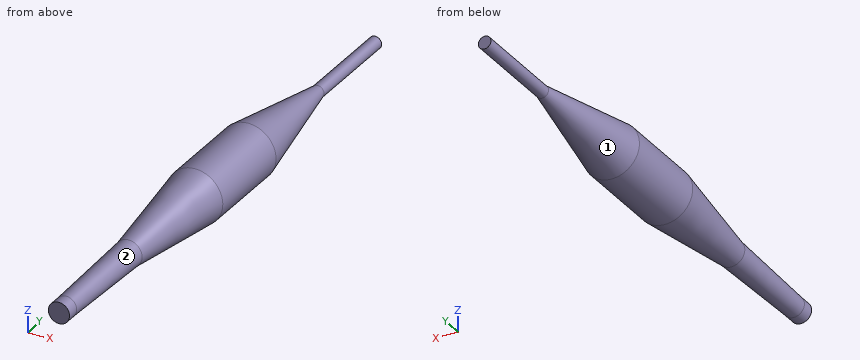
from build123d import *

# Parameters (mm, degrees)
F0_W   = 25
F0_H   = 21
F0_W_2 = 184.9109574539
F0_H_2 = 55
F0_W_3 = 200
F0_H_3 = 12.5


# Not quite as in the source:
# - the program builds the solid bodies; features that only make, move or delete a surface that nothing else refers to are left out


with BuildPart() as f1:
    # F0 (on Right) → F1 (revolve)
    with BuildSketch(Plane.YZ):
        with Locations((12.5, 223.4762815751)):
            Rectangle(F0_W, F0_H)
        Polygon((25, 233.9762815751), (25, 212.9762815751), (242, 212.9762815751), (242, 239.6586265556), align=None)
        Polygon((242, 239.6586265556), (242, 212.9762815751), (344.0616714118, 212.9762815751), (344.0616714118, 252.1902240649), align=None)
        Polygon((344.0616714118, 252.1902240649), (344.0616714118, 212.9762815751), (472.6287925066, 212.9762815751), (472.6287925066, 267.9762815751), align=None)
        with Locations((565.0842712335, 240.4762815751)):
            Rectangle(F0_W_2, F0_H_2)
        Polygon((657.5397499605, 267.9762815751), (657.5397499605, 212.9762815751), (813.5, 212.9762815751), (813.5, 240.4762815751), align=None)
        Polygon((813.5, 240.4762815751), (813.5, 212.9762815751), (898.5692272943, 212.9762815751), (898.5692272943, 225.4762815751), align=None)
        with Locations((998.5692272943, 219.2262815751)):
            Rectangle(F0_W_3, F0_H_3)
    revolve(axis=Axis((0, -32.5, 212.9762815751), (0, -1, 0)))


solid = f1.part
Part model, mm, in its own coordinate system. Face numbers are marked on the shaded views. A direction names the side the tool comes from. Coordinates: 2 decimals unless noted, no trailing zeros. Order: outer loops, then holes, each group sorted by start corner. A loop starts at its lowest first (then second) coordinate and runs counter-clockwise, first axis right, second up. Notation, with made-up numbers: M -10,-10 L 29,-10 A12 ccw 29,13 Z; hole C -29,-8 d7. An arc over 180 degrees is marked long. Use a Markdown table: item, result.
(1) Probe L1, parallel to Z at x = 4, y = 489.5; L2, parallel to X at y = 1023, z = 202.5; L3, parallel to X at y = 628, z = 228. List the from-to ranges inside material, lowest first.
A:
| item | result |
|---|---|
| L1 | z = 158.12 to 267.83 |
| L2 | x = -6.82 to 6.82 |
| L3 | x = -52.91 to 52.91 |
(2) Cut at C-C on y = 927. Write the cut outline in (x, z), then the cut area to 3 significant figures.
A:
| item | result |
|---|---|
| outline | C 0,212.98 d25 |
| area | 491 mm^2 |
(3) Tool access for the marked faces 1 and 2: list every direction of +Z, -Z, +X, -X, +Y, -Y with a clear straight run to the whole face (end or side of a thin tool).
A:
| item | result |
|---|---|
| face 1 | +Y |
| face 2 | -Y |
(4) Cut at A-A on x = 0. Write the cut outline in (y, z), then the cut area to 3 significant figures.
A:
| item | result |
|---|---|
| outline | M 0,191.98 L 25,191.98 L 242,186.29 L 472.63,157.98 L 657.54,157.98 L 898.57,200.48 L 1098.57,200.48 L 1098.57,225.48 L 898.57,225.48 L 657.54,267.98 L 472.63,267.98 L 242,239.66 L 25,233.98 L 0,233.98 Z |
| area | 71,800 mm^2 |
(5) Flat gauge pins, fed straight in: pin 1 (10 mm diameter, centred on x = -13.5, z = 222, fed in from -Y); pin 2 (1.5 mm diameter, centred on x = 26.5, y = 501, fed in from +Z); pin 3 (4 mm diameter, centred on x = -38.5, y = 584.5, fed in from +Z); pin 4 (12 mm diameter, centred on x = -38, y = 362.5, fed in from +Z). Where does each tip first touch, or does it go through?
A:
| item | result |
|---|---|
| pin 1 | stops at y = 0 |
| pin 2 | stops at z = 261.58 |
| pin 3 | stops at z = 254.12 |
| pin 4 | stops at z = 239.46 |
(6) Cut at B-B on y = 535. Write the cut outline in (x, z), then the cut area to 3 significant figures.
A:
| item | result |
|---|---|
| outline | C 0,212.98 d110 |
| area | 9,500 mm^2 |
